Source: three-view drawing plus pictorial views. Frame: mm from the lowest corner of the part. Round coordinates to 2 decimals unless told otherwise and drop trailing zeros. Loops run counter-clockwise (first coordinate to the right, second up) from the corner with the lowest first, then second, coordinate; pieces in that order, holes last. Notation, with made-up numbers: M 77,-2 L 113,-2 A23 ccw 113,15 Z; hole C 47.5,30.5 d4. An arc over 180 degrees is marked long. Answer as a JSON object with one key per item and string values.
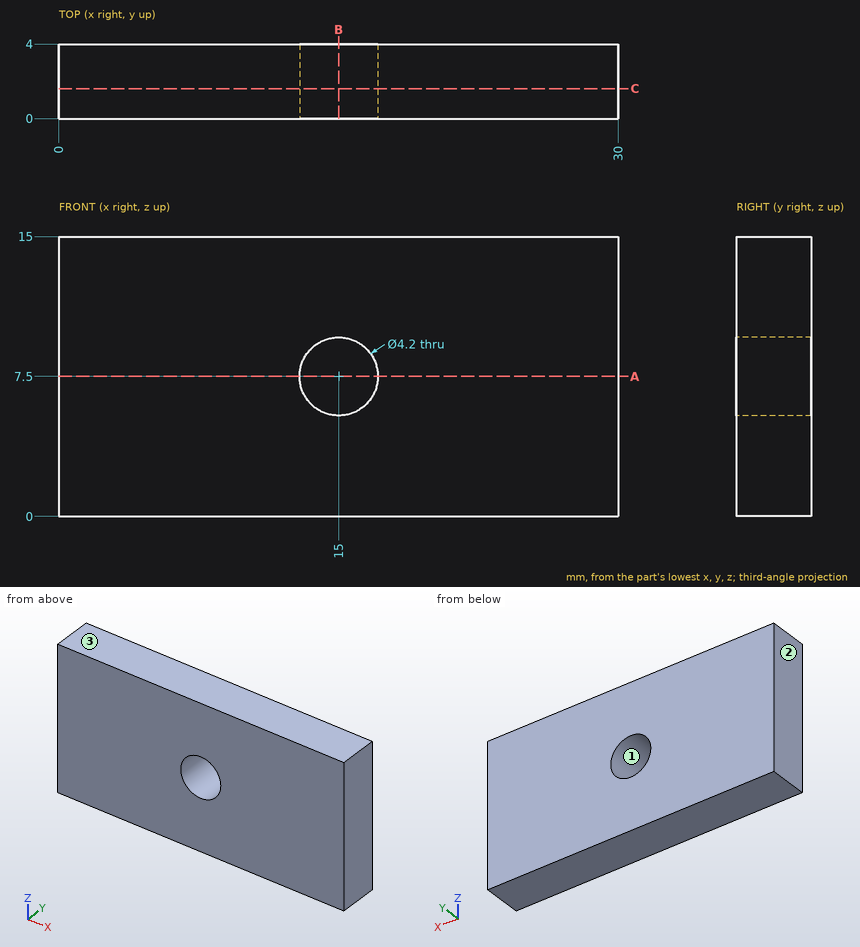
1) Line query: probe 1 along Z at (x, y) = (15, 2.8); probe 2 along X at (y, z) = (2.2, 7.5); probe 3 along X at (y, z) = (3.2, 8.75). Output: solid intervals per line, ascending.
Geometry results:
{"probe 1": "0 to 5.4, 9.6 to 15", "probe 2": "0 to 12.9, 17.1 to 30", "probe 3": "0 to 13.31, 16.69 to 30"}
2) Cut plane A-A on z = 7.5. Return the cut outline in (x, y), and give its area (3 significant figures).
Geometry results:
{"outline": "M 0,0 L 12.9,0 L 12.9,4 L 0,4 Z; M 17.1,0 L 30,0 L 30,4 L 17.1,4 Z", "area": "103 mm2"}
3) Pull-direction query (X, two-part tool) for the marked faces 1, 2 and 3; classes: +X half, -X half, draft (parallel to the pull), parting line (faces both ways), or undercut.
Geometry results:
{"face 1": "undercut", "face 2": "-X half", "face 3": "draft"}
4) Cut plane C-C on y = 1.6. Return the cut outline in (x, z).
Geometry results:
{"outline": "M 0,0 L 30,0 L 30,15 L 0,15 Z; hole C 15,7.5 d4.2"}
5) Cut plane B-B on x = 15. Return the cut outline in (y, z).
Geometry results:
{"outline": "M 0,0 L 4,0 L 4,5.4 L 0,5.4 Z; M 0,9.6 L 4,9.6 L 4,15 L 0,15 Z"}
